Read the model definition and answer for the solid it produces. Units are mm, in the model's axes. Face numbers are marked on the shaded views. Coordinates: 2 decimals unless noted, no trailing zeros. Order: outer loops, then holes, each group sorted by start corner. A loop starts at its lowest first (then second) coordinate and runs counter-clockwise, first axis right, second up.
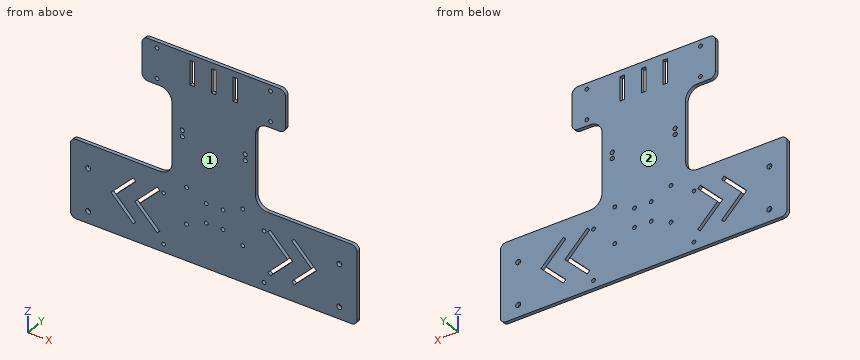
```python
from build123d import *

# Parameters (mm, degrees)
SKETCH_1_W            = 240
SKETCH_1_H            = 65
SKETCH_1_R            = 2.1
EXTRUDE_1_DEPTH       = 3
SKETCH_3_R            = 1.6
CUT_EXTRUDE_1_DEPTH   = 125.359358313
EXTRUDE_2_DEPTH       = 3
FILLET_1_R            = 10
SKETCH_5_R            = 1.6
SKETCH_5_W            = 4
SKETCH_5_H            = 20
CUT_EXTRUDE_2_DEPTH   = 183.524655869
FILLET_2_R            = 10
CUT_EXTRUDE_1_2_DEPTH = 183.524655869
SKETCH_8_R            = 1.75
CUT_EXTRUDE_5_DEPTH   = 183.524655869
SKETCH_9_R            = 1.55
CUT_EXTRUDE_6_DEPTH   = 183.524655869
FILLET_3_R            = 5


with BuildPart() as part:
    # 草图1 → 凸台-拉伸1 (new body)
    # profile 1 of 2: a face of its own
    with BuildSketch(Plane(origin=(0, 0, 0), x_dir=(1, 0, 0), z_dir=(0, 1, 0))):
        Rectangle(SKETCH_1_W, SKETCH_1_H)
        with Locations(Location((105, -12.5, 0), (0, 0, 270))):
            Circle(SKETCH_1_R, mode=Mode.SUBTRACT)
        with Locations(Location((-105, -12.5, 0), (0, 0, 270))):
            Circle(SKETCH_1_R, mode=Mode.SUBTRACT)
        with Locations(Location((-105, 22.5, 0), (0, 0, 270))):
            Circle(SKETCH_1_R, mode=Mode.SUBTRACT)
        with Locations(Location((105, 22.5, 0), (0, 0, 270))):
            Circle(SKETCH_1_R, mode=Mode.SUBTRACT)
    # profile 2 of 2: a face of its own
    with BuildSketch(Plane(origin=(0, 0, 0), x_dir=(1, 0, 0), z_dir=(0, 1, 0))):
        Polygon((-120, 32.5), (-120, -32.5), (-60, -32.5), (20, -32.5), (120, -32.5), (120, 32.5), align=None)
        with Locations(Location((-105, -12.5, 0), (0, 0, 270))):
            Circle(SKETCH_1_R, mode=Mode.SUBTRACT)
        with Locations(Location((105, -12.5, 0), (0, 0, 270))):
            Circle(SKETCH_1_R, mode=Mode.SUBTRACT)
        with Locations(Location((-105, 22.5, 0), (0, 0, 270))):
            Circle(SKETCH_1_R, mode=Mode.SUBTRACT)
        with Locations(Location((105, 22.5, 0), (0, 0, 270))):
            Circle(SKETCH_1_R, mode=Mode.SUBTRACT)
    extrude(amount=EXTRUDE_1_DEPTH)

    # 草图3 → Cut-Extrude 1 (cut, through all)
    with BuildSketch(Plane(origin=(0, 3, 0), x_dir=(1, 0, 0), z_dir=(0, 1, 0))):
        with Locations(Location((-22.773937698, 2.5, 0), (0, 0, 270))):
            Circle(SKETCH_3_R)
        with Locations(Location((24.226062302, 2.5, 0), (0, 0, 90))):
            Circle(SKETCH_3_R)
        with Locations(Location((24.226062302, -27.5, 0), (0, 0, 270))):
            Circle(SKETCH_3_R)
        with Locations(Location((-22.773937698, -27.5, 0), (0, 0, 90))):
            Circle(SKETCH_3_R)
        with Locations(Location((-6.273937698, -4.5, 0), (0, 0, 270))):
            Circle(SKETCH_3_R)
        with Locations(Location((7.726062302, -4.5, 0), (0, 0, 90))):
            Circle(SKETCH_3_R)
        with Locations(Location((7.726062302, -20.5, 0), (0, 0, 270))):
            Circle(SKETCH_3_R)
        with Locations(Location((-6.273937698, -20.5, 0), (0, 0, 90))):
            Circle(SKETCH_3_R)
    extrude(amount=-CUT_EXTRUDE_1_DEPTH, mode=Mode.SUBTRACT)

    # 草图4 → 凸台-拉伸2 (add)
    with BuildSketch(Plane(origin=(0, 0, 0), x_dir=(1, 0, 0), z_dir=(0, 1, 0))):
        Polygon((0, -32.5), (-35, -32.5), (-35, -102.5), (-60, -102.5), (-60, -137.5), (60, -137.5), (60, -102.5), (35, -102.5), (35, -32.5), align=None)
    extrude(amount=EXTRUDE_2_DEPTH)

    # 圆角1
    fillet_1_edges = [part.edges().sort_by_distance(p)[0] for p in [
        (35, 1.5, 32.5),
        (-35, 1.5, 32.5),
    ]]
    fillet(fillet_1_edges, radius=FILLET_1_R)

    # 草图5 → 切除-拉伸2 (cut, through all)
    with BuildSketch(Plane(origin=(0, 3, 0), x_dir=(1, 0, 0), z_dir=(0, 1, 0))):
        with Locations(Location((-47.5, -132.5, 0), (0, 0, 270))):
            Circle(SKETCH_5_R)
        with Locations(Location((47.5, -132.5, 0), (0, 0, 90))):
            Circle(SKETCH_5_R)
        with Locations(Location((-47.5, -107.5, 0), (0, 0, 270))):
            Circle(SKETCH_5_R)
        with Locations(Location((47.5, -107.5, 0), (0, 0, 90))):
            Circle(SKETCH_5_R)
        with Locations((0, -122.5)):
            Rectangle(SKETCH_5_W, SKETCH_5_H)
        with Locations((-18, -122.5)):
            Rectangle(SKETCH_5_W, SKETCH_5_H)
        with Locations((18, -122.5)):
            Rectangle(SKETCH_5_W, SKETCH_5_H)
    extrude(amount=-CUT_EXTRUDE_2_DEPTH, mode=Mode.SUBTRACT)

    # 圆角2
    fillet_2_edges = [part.edges().sort_by_distance(p)[0] for p in [
        (35, 1.5, 102.5),
        (-35, 1.5, 102.5),
    ]]
    fillet(fillet_2_edges, radius=FILLET_2_R)

    # 草图7 → Cut-Extrude 1 2 (cut, through all)
    with BuildSketch(Plane(origin=(0, 3, 0), x_dir=(1, 0, 0), z_dir=(0, 1, 0))):
        Polygon((-45.148639148, -16.617009358), (-61.765648506, 0), (-45.148639148, 16.617009358), (-47.269959491, 18.738329701), (-66.008289193, 0), (-47.269959491, -18.738329701), align=None)
        Polygon((-65.148639148, -16.617009358), (-81.765648506, 0), (-65.148639148, 16.617009358), (-67.269959491, 18.738329701), (-86.008289193, 0), (-67.269959491, -18.738329701), align=None)
        Polygon((65.148639148, 16.617009358), (81.765648506, 0), (65.148639148, -16.617009358), (67.269959491, -18.738329701), (86.008289193, 0), (67.269959491, 18.738329701), align=None)
        Polygon((45.148639148, 16.617009358), (61.765648506, 0), (45.148639148, -16.617009358), (47.269959491, -18.738329701), (66.008289193, 0), (47.269959491, 18.738329701), align=None)
    extrude(amount=-CUT_EXTRUDE_1_2_DEPTH, mode=Mode.SUBTRACT)

    # 草图8 → 切除-拉伸5 (cut, through all)
    with BuildSketch(Plane(origin=(0, 3, 0), x_dir=(1, 0, 0), z_dir=(0, 1, 0))):
        with Locations(Location((-26.316332853, -68, 0), (0, 0, 270))):
            Circle(SKETCH_8_R)
        with Locations(Location((-26.316332853, -73, 0), (0, 0, 90))):
            Circle(SKETCH_8_R)
        with Locations(Location((26.316332853, -73, 0), (0, 0, 270))):
            Circle(SKETCH_8_R)
        with Locations(Location((26.316332853, -68, 0), (0, 0, 90))):
            Circle(SKETCH_8_R)
    extrude(amount=-CUT_EXTRUDE_5_DEPTH, mode=Mode.SUBTRACT)

    # 草图9 → 切除-拉伸6 (cut, through all)
    with BuildSketch(Plane(origin=(0, 3, 0), x_dir=(1, 0, 0), z_dir=(0, 1, 0))):
        with Locations(Location((-42, 26, 0), (0, 0, 270))):
            Circle(SKETCH_9_R)
        with Locations(Location((-42, -16, 0), (0, 0, 270))):
            Circle(SKETCH_9_R)
        with Locations(Location((42, -16, 0), (0, 0, 90))):
            Circle(SKETCH_9_R)
        with Locations(Location((42, 26, 0), (0, 0, 90))):
            Circle(SKETCH_9_R)
    extrude(amount=-CUT_EXTRUDE_6_DEPTH, mode=Mode.SUBTRACT)

    # 圆角3
    fillet_3_edges = [part.edges().sort_by_distance(p)[0] for p in [
        (-120, 1.5, 32.5),
        (-120, 1.5, -32.5),
        (120, 1.5, -32.5),
        (120, 1.5, 32.5),
        (-60, 1.5, 137.5),
        (60, 1.5, 137.5),
        (60, 1.5, 102.5),
        (-60, 1.5, 102.5),
    ]]
    fillet(fillet_3_edges, radius=FILLET_3_R)


solid = part.part
```
1) Flat-ended cylindrical pins translate along their axes: pin 1 Ø3.5 at (x, z) = (105, 12.5) entering from -Y; pin 2 Ø1 at (x, y) = (73, 1) entering from +Z; pin 3 Ø1 at (x, y) = (-57, 1.5) entering from +Z; pin 4 Ø1.5 at (y, z) = (2, 127.5) entering from -X. Find the tip coordinate at first contact, or state that the pin passes through.
A:
pin 1: passes through
pin 2: stops at z = 32.5
pin 3: stops at z = 137.27
pin 4: stops at x = -60
2) A cutting plane is placed at C-C, the plane y = 0.5. State how many separate pieces and enclosed holes the cut face has, and give its area (3 significant figures).
A:
separate pieces: 1
enclosed holes: 31
area: 23,700 mm2
3) Determine the mould class of the marked faces 1 and 2 for opening direction Y: pulls with the +Y half, pulls with the -Y half, needs draft (parallel to the pull), parting line crosses it, or undercut.
A:
face 1: pulls with the -Y half
face 2: pulls with the +Y half
4) A cutting plane is placed at A-A, the plane z = 126.5. Determine the outline of the cut face in (x, y).
A:
outline: (-60, 0) - (-20, 0) - (-20, 3) - (-60, 3) - close; (-16, 0) - (-2, 0) - (-2, 3) - (-16, 3) - close; (2, 0) - (16, 0) - (16, 3) - (2, 3) - close; (20, 0) - (60, 0) - (60, 3) - (20, 3) - close
5) A cutting plane is placed at B-B, the plane z = -8. Determine the outline of the cut face in (x, y), and give its area (3 significant figures).
A:
outline: (-120, 0) - (-78.01, 0) - (-78.01, 3) - (-120, 3) - close; (-73.77, 0) - (-58.01, 0) - (-58.01, 3) - (-73.77, 3) - close; (-53.77, 0) - (53.77, 0) - (53.77, 3) - (-53.77, 3) - close; (58.01, 0) - (73.77, 0) - (73.77, 3) - (58.01, 3) - close; (78.01, 0) - (120, 0) - (120, 3) - (78.01, 3) - close
area: 669 mm2
6) A cutting plane is placed at D-D, the plane z = 80. Determine the outline of the cut face in (x, y).
A:
outline: (-35, 0) - (35, 0) - (35, 3) - (-35, 3) - close
7) Straight lines are drawn through the part: line 1 (X direction, y = 1.7, z = 20.5); line 2 (X direction, y = 1.4, z = -26); line 3 (X direction, y = 1, z = 118.5). For each, find the intervals that lie inside material, in ascending order.
A:
line 1: x = -120 to -7.87, -4.67 to 6.13, 9.33 to 120
line 2: x = -120 to -43.55, -40.45 to 40.45, 43.55 to 120
line 3: x = -60 to -20, -16 to -2, 2 to 16, 20 to 60
